Check sheet for the drawn part. Datum: minimum x, y, z corner. Units: mm. Give positions to 0.01 mm unless a question says otherwise; leave off trailing zeros. Write each loop counter-clockwise with the first axis right and the second up, starting at its lowest first coordinate (ties: lowest second). Pieces come first, ordered by that corner, then holes.
(1) Thickness scan on line 1 along X through (y, z) = (207, 4.5); line 2 along Z through (x, y) = (92, 24.5); line 3 along X through (y, z) = (63, 5). Record the ranges inside material, lowest first.
(2) Cross-section at B-B (z = 6). Record the boundary of the cut face in (x, y), and give its area (3 significant figures).
(3) Cross-section at A-A (x = 94.5). Record the boundary of the cut face in (y, z).
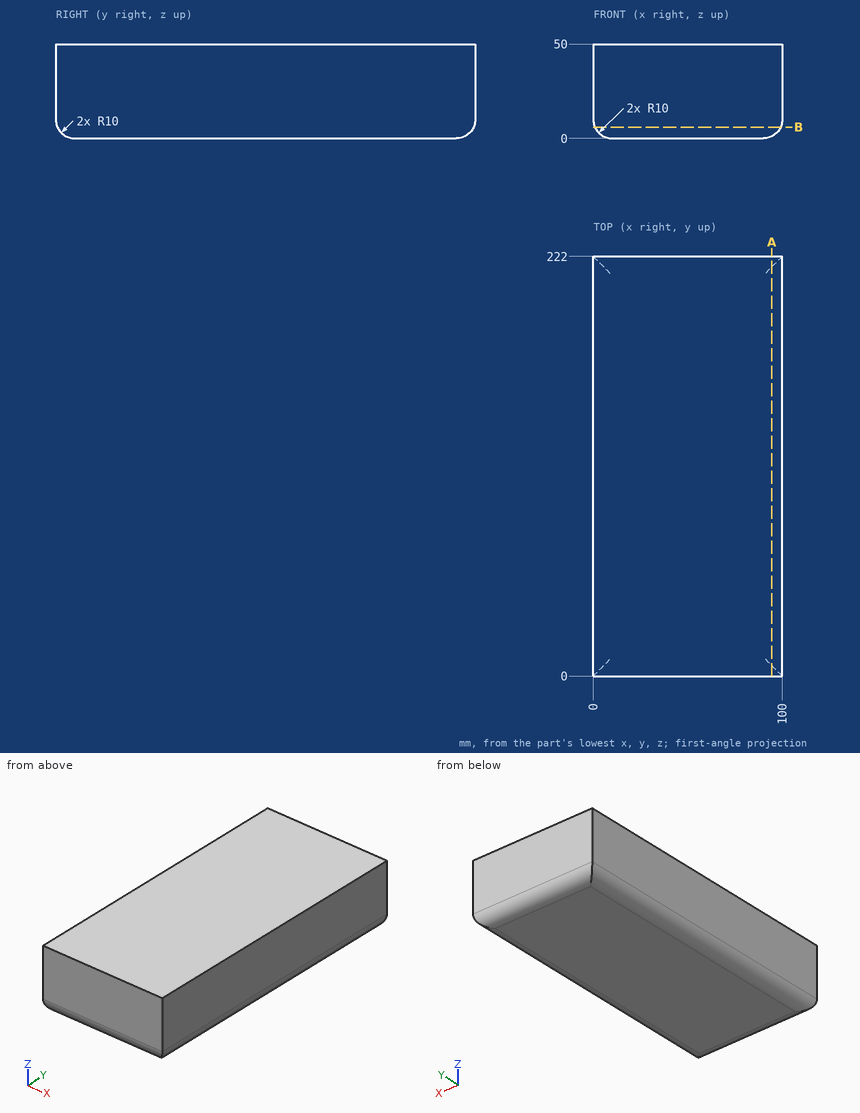
Reply:
1. line 1: x = 1.65 to 98.35
1. line 2: z = 0.2 to 50
1. line 3: x = 1.34 to 98.66
2. outline: (0.83, 0.83) - (99.17, 0.83) - (99.17, 221.17) - (0.83, 221.17) - close
2. area: 21,700 mm2
3. outline: (0, 10) arc R10 ccw to (5.5, 1.07) - (216.5, 1.07) arc R10 ccw to (222, 10) - (222, 50) - (0, 50) - close
